Check sheet for the modelled part. Datum: model origin and axes. Units: mm. A direction names the side the tool comes from. Round coordinates to 2 decimals unless told otherwise and drop trailing zeros. Write each loop counter-clockwise with the first axis right and the second up, starting at its lowest first coordinate (ties: lowest second). Pieces come first, ordered by that corner, then holes. Notation, with made-up numbers: (-21.75, 53.25) - (10.25, 53.25) arc R13 ccw to (10.25, 77.25) - close; hole circle Ø7 at (-25.5, 84). An arc over 180 degrees is marked (long way). Use one line per item in the form item = value. Start each with the question number.
1) Section check A-A (y = 68.5). Record the boundary of the cut face in (x, z).
2) Section check B-B (z = 11.5). Record the boundary of the cut face in (x, y).
3) Draft check along Z on faces 1 (the face through (9, 100, 5)), 2 (the face through (-25.668, 54.23, 10.458)), 3 (the face through (25.668, 54.23, -10.458)). Enter one of: +Z half, -Z half, draft (parallel to the pull), parting line (faces both ways), or undercut.
4) Gauge pin test, flat ends, axial feed: P1, Ø2, axis at y = 40.5, z = -19.5, coming from the +X side; P2, Ø4, axis at y = 57.5, z = 24, coming from the +X side; P3, Ø18, axis at x = 0, z = 0, coming from the -Y side; P4, Ø2, axis at y = 79, z = 18.5, coming from the +X side. Record the tip position at first contact, or that the pin passes through.
5) Section check D-D (z = 26.5). Record the boundary of the cut face in (x, y).
6) Section check C-C (x = -17). Record the boundary of the cut face in (y, z).
7) Scan lines: probe 1 along X at (y, z) = (104, 0); probe 2 along X at (y, z) = (25, 0); probe 3 along Z at (x, y) = (-16.5, 56.5). Record each from-to range of solid material in increasing order.
8) Set-up check for faces 4 (the face through (-19.524, 49.3, 4.336)), 5 (the face through (25.545, 54.23, 10.755)): record each of +Z, -Z, +X, -X, +Y, -Y from which the full face is reachable in a straight line by a thin tool's end or side.
from build123d import *

# Parameters (mm, degrees)
BOSS_EXTRUDE1_DEPTH = 110
SKETCH2_R           = 10
CUT_EXTRUDE1_DEPTH  = 110
SKETCH3_R           = 20
CUT_EXTRUDE2_DEPTH  = 100


with BuildPart() as part:
    # Sketch1 → Boss-Extrude1 (new body)
    with BuildSketch(Plane(origin=(0, 0, 0), x_dir=(1, 0, 0), z_dir=(0, 1, 0))):
        Polygon((30, 0), (21.213203436, 21.213203436), (0, 30), (-21.213203436, 21.213203436), (-30, 0), (-21.213203436, -21.213203436), (0, -30), (21.213203436, -21.213203436), align=None)
    extrude(amount=BOSS_EXTRUDE1_DEPTH)

    # Sketch2 → Cut-Extrude1 (cut)
    with BuildSketch(Plane(origin=(0, 110, 0), x_dir=(1, 0, 0), z_dir=(0, 1, 0))):
        with Locations(Location((0, 0, 0), (0, 0, 270))):
            Circle(SKETCH2_R)
    extrude(amount=-CUT_EXTRUDE1_DEPTH, mode=Mode.SUBTRACT)

    # Sketch3 → Cut-Extrude2 (cut)
    with BuildSketch(Plane.XZ):
        with Locations(Location((0, 0, 0), (0, 0, 270))):
            Circle(SKETCH3_R)
    extrude(amount=-CUT_EXTRUDE2_DEPTH, mode=Mode.SUBTRACT)


solid = part.part
Results are:
q1.outline = (-30, 0) - (-21.21, -21.21) - (0, -30) - (21.21, -21.21) - (30, 0) - (21.21, 21.21) - (0, 30) - (-21.21, 21.21) - close; hole circle Ø40 at (0, 0)
q2.outline = (-25.24, 0) - (-16.36, 0) - (-16.36, 100) - (16.36, 100) - (16.36, 0) - (25.24, 0) - (25.24, 110) - (-25.24, 110) - close
q3.face_1 = undercut
q3.face_2 = +Z half
q3.face_3 = -Z half
q4.P1 = 22.34
q4.P2 = 19.31
q4.P3 = through
q4.P4 = 22.75
q5.outline = (-8.45, 0) - (8.45, 0) - (8.45, 110) - (-8.45, 110) - close
q6.outline = (0, -22.96) - (110, -22.96) - (110, 22.96) - (0, 22.96) - (0, 10.54) - (100, 10.54) - (100, -10.54) - (0, -10.54) - close
q7.probe_1 = -30 to -10, 10 to 30
q7.probe_2 = -30 to -20, 20 to 30
q7.probe_3 = -23.17 to -11.3, 11.3 to 23.17
q8.face_4 = -Y
q8.face_5 = +Z, +X, +Y, -Y
